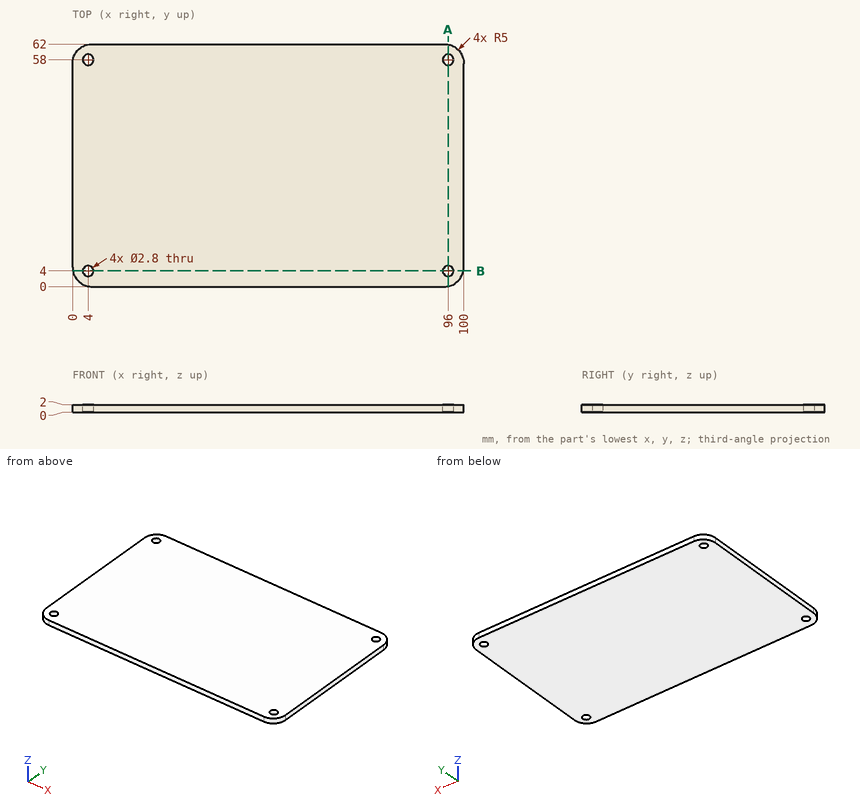
Design review of the part shown in the three views and the two pictorial views. Dimensions are in mm from the part's minimum x, y and z. Round coordinates to 2 decimals unless told otherwise and drop trailing zeros. Loops run counter-clockwise (first coordinate to the right, second up) from the corner with the lowest first, then second, coordinate; pieces in that order, holes last. Notation, with made-up numbers: (86, 73.5) - (93, 73.5) arc R10 ccw to (93, 88.5) - close; hole circle Ø9 at (45.5, 69.25). An arc over 180 degrees is marked (long way). Use one line per item in the form item = value.
1) Clearance check with a flat-ended pin moving along its axis: P1, Ø2, axis at x = 96, y = 4, coming from the -Z side. State where the tip first meets the part, or that it passes through.
Solutions:
P1 = through
2) We need section A-A on x = 96. Write out the cut boundary in (y, z), then the cut area to 3 significant figures.
Solutions:
outline = (0.1, 0) - (2.6, 0) - (2.6, 2) - (0.1, 2) - close; (5.4, 0) - (56.6, 0) - (56.6, 2) - (5.4, 2) - close; (59.4, 0) - (61.9, 0) - (61.9, 2) - (59.4, 2) - close
area = 112 mm2
3) We need section B-B on y = 4. Write out the cut boundary in (x, z), then the cut area to 3 significant figures.
Solutions:
outline = (0.1, 0) - (2.6, 0) - (2.6, 2) - (0.1, 2) - close; (5.4, 0) - (94.6, 0) - (94.6, 2) - (5.4, 2) - close; (97.4, 0) - (99.9, 0) - (99.9, 2) - (97.4, 2) - close
area = 188 mm2
4) Wall thickness on probe 1 along X at (y, z) = (57, 1.1); probe 2 along X at (y, z) = (4.5, 0.55); probe 3 along Y at (x, z) = (96, 1.2): over which ranges is each line inside the solid? List them lowest first.
Solutions:
probe_1 = 0 to 3.02, 4.98 to 95.02, 96.98 to 100
probe_2 = 0.03 to 2.69, 5.31 to 94.69, 97.31 to 99.97
probe_3 = 0.1 to 2.6, 5.4 to 56.6, 59.4 to 61.9
